Autodesk Inventor part; units mm, degrees
ref_plane "YZ Plane" through (0, 0, 0) normal (1, 0, 0) x (0, 1, 0)
ref_plane "XZ Plane" through (0, 0, 0) normal (0, 1, 0) x (-1, 0, 0)
ref_plane "XY Plane" through (0, 0, 0) normal (0, 0, 1) x (1, 0, 0)
sketch "Sketch1" plane through (0, 0, 0) normal (0, 1, 0) x (-1, 0, 0)
  line L0 (-20, 25) -> (20, 25)
  line L1 (20, 25) -> (20, -25)
  line L2 (20, -25) -> (-20, -25)
  line L3 (-20, -25) -> (-20, 25)
  line L4 (-20, 25) -> (20, -25) construction
  line L5 (20, 25) -> (-20, -25) construction
  line L6 (17, 14) -> (7, 14) construction
  arc A0 (7, 14) -> (4, 11) centre (7, 11) ccw construction
  line L7 (4, 11) -> (4, -11) construction
  arc A1 (4, -11) -> (7, -14) centre (7, -11) ccw construction
  line L8 (7, -14) -> (17, -14) construction
  arc A2 (17, -14) -> (20, -11) centre (17, -11) ccw construction
  line L9 (20, -11) -> (20, 11) construction
  arc A3 (20, 11) -> (17, 14) centre (17, 11) ccw construction
  circle A4 centre (17.5, -0.5) radius 2 construction
  circle A5 centre (17, 11) radius 1.7 construction
  circle A6 centre (7, -11) radius 1.7 construction
  line L10 (4, 0) -> (20, 0) construction
  line L11 (17, -14) -> (7, -14) construction
  arc A7 (4, -11) -> (7, -14) centre (7, -11) ccw construction
  line L12 (4, -11) -> (4, 11) construction
  arc A8 (7, 14) -> (4, 11) centre (7, 11) ccw construction
  line L13 (7, 14) -> (17, 14) construction
  arc A9 (20, 11) -> (17, 14) centre (17, 11) ccw construction
  line L14 (20, 11) -> (20, -11) construction
  arc A10 (17, -14) -> (20, -11) centre (17, -11) ccw construction
  circle A11 centre (17.5, 0.5) radius 2 construction
  circle A12 centre (17, -11) radius 1.7
  circle A13 centre (7, 11) radius 1.7
  line L15 (20, 0) -> (-20, 0) construction
  line L16 (0, 25) -> (0, -25) construction
  line L17 (-10, 25) -> (-10, -25) construction
  circle A14 centre (-10, 15) radius 2
  circle A15 centre (-10, -15) radius 2
  point P0 (0, 0)
  point P1 (12, 0)
  dimension "d0" = 40
  dimension "d1" = 50
  dimension "d5" = 10
  dimension "d6" = 4
  dimension "d7" = 4
  dimension "d8" = 10
  dimension "d9" = 10
extrude "Extrusion2" add sketch "Sketch1" along normal blind 5
fillet "Fillet2" radius 4 4 edges at (20, 2.5, -25) (20, 2.5, 25) (-20, 2.5, -25) (-20, 2.5, 25)
properties part number "Soporte_Final_Carrera"
Design review of the part built by this model. Coordinates are the model's own, in mm. Round coordinates to 2 decimals unless told otherwise and drop trailing zeros. Write each loop counter-clockwise with the first axis right and the second up, starting at its lowest first coordinate (ties: lowest second). Pieces come first, ordered by that corner, then holes.
Item 1: The part is to be moulded in two halves that separate along Z. For faces 1 (the flat face through (-20, 2, 0)), 2 (the cylindrical face through (-18.57, 2.46, -10.35)), 3 (the cylindrical face through (18.797, 2.535, 23.859)), say which applies: +Z half, -Z half, draft (parallel to the pull), parting line (faces both ways), or undercut.
Item 2: We need section A-A on x = -7. Write out the cut boundary in (y, z), and give its area (3 significant figures).
Item 3: Clearance check with flat-ended pins moving along their axes: pin 1 Ø8 at (x, z) = (-6.5, 10.5) entering from +Y; pin 2 Ø2.5 at (x, z) = (-17, -11) entering from -Y (3 decimals). State where each tip first meets the part, or that it passes through.
Item 4: For probe 1 along Z at (x, y) = (10, 2.4); probe 2 along Z at (x, y) = (-7, 2.25); probe 3 along Z at (x, y) = (9, 3.15), list the stretches that pass through material, from the lowest coordinate up.
Item 5: We need section B-B on z = 11. Write out the cut boundary in (x, y), and give its area (3 significant figures).
Item 6: We need section D-D on x = 10. Write out the cut boundary in (y, z).
Item 7: We need section C-C on y = 3.1. Write out the cut boundary in (x, z).
Returned:
1. face 1: draft
1. face 2: undercut
1. face 3: +Z half
2. outline: (0, -25) - (5, -25) - (5, 9.3) - (0, 9.3) - close; (0, 12.7) - (5, 12.7) - (5, 25) - (0, 25) - close
2. area: 233 mm2
3. pin 1: stops at y = 5
3. pin 2: passes through
4. probe 1: z = -25 to -17, -13 to 13, 17 to 25
4. probe 2: z = -25 to 9.3, 12.7 to 25
4. probe 3: z = -25 to -16.73, -13.27 to 13.27, 16.73 to 25
5. outline: (-20, 0) - (-8.7, 0) - (-8.7, 5) - (-20, 5) - close; (-5.3, 0) - (20, 0) - (20, 5) - (-5.3, 5) - close
5. area: 183 mm2
6. outline: (0, -25) - (5, -25) - (5, -17) - (0, -17) - close; (0, -13) - (5, -13) - (5, 13) - (0, 13) - close; (0, 17) - (5, 17) - (5, 25) - (0, 25) - close
7. outline: (-20, -21) arc R4 ccw to (-16, -25) - (16, -25) arc R4 ccw to (20, -21) - (20, 21) arc R4 ccw to (16, 25) - (-16, 25) arc R4 ccw to (-20, 21) - close; hole circle Ø3.4 at (-17, -11); hole circle Ø3.4 at (-7, 11); hole circle Ø4 at (10, -15); hole circle Ø4 at (10, 15)
